Could you check a few things on this model? Use its own coordinates, in mm. A direction names the side the tool comes from. Round coordinates to 2 decimals unless told otherwise and drop trailing zeros. Loops run counter-clockwise (first coordinate to the right, second up) from the corner with the lowest first, then second, coordinate; pieces in that order, holes last. Notation, with made-up numbers: (-2.75, 87) - (31.25, 87) arc R10 cw to (31.25, 100) - close; hole circle Ø1 at (-23.75, 85). An arc over 180 degrees is marked (long way). Answer as CSV lines item,"result". Start each with the question number.
1) Suppose I cut it at D-D, the plane x = 2.25. Write out the boundary of the cut face in (y, z).
2) Suppose I cut it at B-B, the plane z = 0. Write out the boundary of the cut face in (x, y), then the cut area to 3 significant figures.
3) Which directions (+Z, -Z, +X, -X, +Y, -Y) give clear straight access to the entire face, cutting with the end or side of a thin tool? Please do faces 1 (the face through (0, 8, 0)), 2 (the face through (-4, 2, -4)), 3 (the face through (0, -6, 5.9)).
4) Suppose I cut it at A-A, the plane x = 0. Write out the boundary of the cut face in (y, z).
5) Suppose I cut it at C-C, the plane y = -3. Write out the boundary of the cut face in (x, z).
6) Please list where these lines run through material, in increasing order: line 1 along Y through (x, z) = (-4.5, 4.25); line 2 along X through (y, z) = (-2, -2.5); line 3 along X through (y, z) = (3, 1).
7) I'm going to push flat-ended pins straight in: pin 1 Ø3 at (x, z) = (-5.5, 2) entering from +Y; pin 2 Ø1 at (x, y) = (3, -3) entering from -Z; pin 3 Ø1.8 at (x, y) = (0, -6) entering from +Z. Where does each tip first touch, or does it pass through?
```python
from build123d import *

# Parameters (mm, degrees)
SKIZZE2_R                       = 7
AUFSATZ_LINEAR_AUSTRAGEN2_DEPTH = 2
SKIZZE4_R                       = 5.5
AUFSATZ_LINEAR_AUSTRAGEN3_DEPTH = 6
SKIZZE5_R                       = 5.4
AUFSATZ_LINEAR_AUSTRAGEN4_DEPTH = 6.7
SKIZZE7_W                       = 1.619965962
SKIZZE7_H                       = 1
AUFSATZ_LINEAR_AUSTRAGEN5_DEPTH = 2


with BuildPart() as part:
    # Skizze2 → Aufsatz-Linear austragen2 (new body)
    with BuildSketch(Plane(origin=(0, 0, 0), x_dir=(1, 0, 0), z_dir=(0, 1, 0))):
        with Locations(Location((0, 0, 0), (0, 0, 270))):
            Circle(SKIZZE2_R)
    extrude(amount=AUFSATZ_LINEAR_AUSTRAGEN2_DEPTH)

    # Skizze4 → Aufsatz-Linear austragen3 (add)
    with BuildSketch(Plane(origin=(0, 2, 0), x_dir=(1, 0, 0), z_dir=(0, 1, 0))):
        with Locations(Location((0, 0, 0), (0, 0, 270))):
            Circle(SKIZZE4_R)
    extrude(amount=AUFSATZ_LINEAR_AUSTRAGEN3_DEPTH)

    # Skizze5 → Aufsatz-Linear austragen4 (add)
    with BuildSketch(Plane(origin=(0, 0, 0), x_dir=(-1, 0, 0), z_dir=(0, -1, 0))):
        with Locations(Location((0, 0, 0), (0, 0, 90))):
            Circle(SKIZZE5_R)
    extrude(amount=AUFSATZ_LINEAR_AUSTRAGEN4_DEPTH)

    # Skizze7 → Aufsatz-Linear austragen5 (add)
    with BuildSketch(Plane.XZ.offset(6.7)):
        with Locations((0, 5.4)):
            Rectangle(SKIZZE7_W, SKIZZE7_H)
    extrude(amount=-AUFSATZ_LINEAR_AUSTRAGEN5_DEPTH)


solid = part.part
```
Filled sheet:
1,outline,"(-6.7, -4.91) - (0, -4.91) - (0, -6.63) - (2, -6.63) - (2, -5.02) - (8, -5.02) - (8, 5.02) - (2, 5.02) - (2, 6.63) - (0, 6.63) - (0, 4.91) - (-6.7, 4.91) - close"
2,outline,"(-7, 0) - (-5.4, 0) - (-5.4, -6.7) - (5.4, -6.7) - (5.4, 0) - (7, 0) - (7, 2) - (5.5, 2) - (5.5, 8) - (-5.5, 8) - (-5.5, 2) - (-7, 2) - close"
2,area,"166 mm²"
3,face 1,"+Z, -Z, +X, -X, +Y"
3,face 2,"+Y"
3,face 3,"+Z, +X, -X, -Y"
4,outline,"(-6.7, -5.4) - (0, -5.4) - (0, -7) - (2, -7) - (2, -5.5) - (8, -5.5) - (8, 5.5) - (2, 5.5) - (2, 7) - (0, 7) - (0, 5.4) - (-4.7, 5.4) - (-4.7, 5.9) - (-6.7, 5.9) - close"
5,outline,"circle Ø10.8 at (0, 0)"
6,line 1,"0 to 2"
6,line 2,"-4.79 to 4.79"
6,line 3,"-5.41 to 5.41"
7,pin 1,"y = 8"
7,pin 2,"z = -4.79"
7,pin 3,"z = 5.9"
